```python
from build123d import *

# Parameters (mm, degrees)
RESSALTO_EXTRUS_O1_DEPTH                  = 110
ESBO_O2_W                                 = 6
ESBO_O2_H                                 = 18
CORTE_EXTRUS_O1_DEPTH                     = 10.53
BROCA_DE_ROSQUEAR_PARA_TARRAXA_DE_M10X1_D = 8.5


with BuildPart() as part:
    # Esboço1 → Ressalto-extrusão1 (new body)
    with BuildSketch(Plane.XY):
        with BuildLine():
            Line((9.53, 0), (45, 0))
            Line((45, 0), (45, 9.53))
            Line((45, 9.53), (14.295, 9.53))
            ThreePointArc((14.295, 9.53), (10.925636188, 10.925636188), (9.53, 14.295))
            Line((9.53, 14.295), (9.53, 39.53))
            Line((9.53, 39.53), (0, 39.53))
            Line((0, 39.53), (0, 9.53))
            ThreePointArc((0, 9.53), (2.791272375, 2.791272375), (9.53, 0))
        make_face()
    extrude(amount=RESSALTO_EXTRUS_O1_DEPTH)

    # Esboço2 → Corte-extrusão1 (cut, through all)
    with BuildSketch(Plane(origin=(9.53, 0, 0), x_dir=(0, 0, -1), z_dir=(1, 0, 0))):
        with Locations((-7.65, 30.53)):
            Rectangle(ESBO_O2_W, ESBO_O2_H)
        with Locations((-97.65, 30.53)):
            Rectangle(ESBO_O2_W, ESBO_O2_H)
        with Locations((-77.65, 30.53)):
            Rectangle(ESBO_O2_W, ESBO_O2_H)
        with Locations((-67.65, 30.53)):
            Rectangle(ESBO_O2_W, ESBO_O2_H)
        with Locations((-57.65, 30.53)):
            Rectangle(ESBO_O2_W, ESBO_O2_H)
        with Locations((-47.65, 30.53)):
            Rectangle(ESBO_O2_W, ESBO_O2_H)
        with Locations((-37.65, 30.53)):
            Rectangle(ESBO_O2_W, ESBO_O2_H)
        with Locations((-27.65, 30.53)):
            Rectangle(ESBO_O2_W, ESBO_O2_H)
        with Locations((-17.65, 30.53)):
            Rectangle(ESBO_O2_W, ESBO_O2_H)
        with Locations((-87.65, 30.53)):
            Rectangle(ESBO_O2_W, ESBO_O2_H)
    extrude(amount=-CORTE_EXTRUS_O1_DEPTH, mode=Mode.SUBTRACT)

    # Broca de rosquear para tarraxa de M10x1.51 (through all)
    with Locations(Plane(origin=(32.38, 9.53, 15), x_dir=(1, 0, 0), z_dir=(0, 1, 0))):
        with Locations((0, 0), (0, -40), (0, -80)):
            Hole(BROCA_DE_ROSQUEAR_PARA_TARRAXA_DE_M10X1_D / 2)


solid = part.part
```
Source: CAD feature listing. Evaluate the final solid. Frame: model axes, mm. A direction names the side the tool comes from. Coordinates: 2 decimals unless noted, no trailing zeros. Loops run counter-clockwise (first coordinate to the right, second up) from the corner with the lowest first, then second, coordinate; pieces in that order, holes last. Notation, with made-up numbers: M -31.5,-0.75 L -25.5,-0.75 A21 ccw -25.5,13.25 Z; hole C 33,15 d6. An arc over 180 degrees is marked long. Use a Markdown table: item, result. Add a question column.
Q1. Section query C-C, the plane y = 5. Return loops of the section in (x, z).
Q2. Draft query along X for faces 1 (the flat face through (45, 5, 54)), 2 (the flat face through (5, 21.53, 98)), 3 (the cylindrical face through (33.3, 4.7, 19.15)), 4 (the flat face through (0, 21, 66)). Return one class per face: pulls with the +X half, pulls with the -X half, needs draft (parallel to the pull), parting line crosses it, or undercut.
Q3. Section query B-B, the plane x = 32.38. Return loops of the section in (y, z), and give its area (3 significant figures).
Q4. Section query D-D, the plane z = 73. Return loops of the section in (x, y) (3 decimals), and give its area (3 significant figures).
Q5. Section query A-A, the plane z = 93. Return loops of the section in (x, y) (3 decimals), and give its area (3 significant figures).
Q6. Access query for faces 5 (the flat face through (5, 21.53, 48)), 6 (the flat face through (17, 7, 0)). Directions: +Z, -Z, +X, -X, +Y, -Y. A direction counts if a zero-diameter tool reaches every point of the face in a straight line with its end or side. Return the directions, or none.
Q7. First-contact query: pin 1 (24.5 mm diameter, centred on x = 26, z = 71.5, fed in from +Y); pin 2 (10 mm diameter, centred on x = 32.38, z = 55, fed in from +Y); pin 3 (20 mm diameter, centred on y = 33, z = 40, fed in from +X). Flat tips, straight axial feed; report the tip coordinate or a pass-through.
Q8. Material intervals for L1, parallel to Z at x = 32, y = 5; L2, parallel to Y at x = 25.5, z = 48, sorted ascending.
Result:
| question | item | result |
|---|---|---|
| 1 | outline | M 1.15,0 L 45,0 L 45,110 L 1.15,110 Z; hole C 32.38,15 d8.5; hole C 32.38,55 d8.5; hole C 32.38,95 d8.5 |
| 2 | face 1 | pulls with the +X half |
| 2 | face 2 | needs draft |
| 2 | face 3 | undercut |
| 2 | face 4 | pulls with the -X half |
| 3 | outline | M 0,0 L 9.53,0 L 9.53,10.75 L 0,10.75 Z; M 0,19.25 L 9.53,19.25 L 9.53,50.75 L 0,50.75 Z; M 0,59.25 L 9.53,59.25 L 9.53,90.75 L 0,90.75 Z; M 0,99.25 L 9.53,99.25 L 9.53,110 L 0,110 Z |
| 3 | area | 805 mm2 |
| 4 | outline | M 0,9.53 A9.53 ccw 9.53,0 L 45,0 L 45,9.53 L 14.295,9.53 A4.765 cw 9.53,14.295 L 9.53,39.53 L 0,39.53 Z |
| 4 | area | 700 mm2 |
| 5 | outline | M 0,9.53 A9.53 ccw 9.53,0 L 28.63,0 L 28.63,9.53 L 14.295,9.53 A4.765 cw 9.53,14.295 L 9.53,39.53 L 0,39.53 Z; M 36.13,0 L 45,0 L 45,9.53 L 36.13,9.53 Z |
| 5 | area | 629 mm2 |
| 6 | face 5 | +X, -X, +Y |
| 6 | face 6 | -Z, +X, -X, +Y, -Y |
| 7 | pin 1 | stops at y = 9.56 |
| 7 | pin 2 | stops at y = 9.53 |
| 7 | pin 3 | stops at x = 9.53 |
| 8 | L1 | z = 0 to 10.77, 19.23 to 50.77, 59.23 to 90.77, 99.23 to 110 |
| 8 | L2 | y = 0 to 9.53 |
